Geometry: final body of the model. Coordinates: model frame, mm. A direction names the side the tool comes from. Round coordinates to 2 decimals unless told otherwise and drop trailing zeros. Order: outer loops, then holes, each group sorted by start corner. A loop starts at its lowest first (then second) coordinate and runs counter-clockwise, first axis right, second up. Notation, with made-up numbers: (77, 79.5) -> (132, 79.5) arc R23 cw to (132, 110.5) -> close; hole circle Ø3 at (62.5, 38.5). An arc over 180 degrees is marked (long way). Put each result on its own line as item: value.
```python
from build123d import *

# Parameters (mm, degrees)
SKETCH_W             = 14
SKETCH_H             = 6
PAD_DEPTH            = 4.8
THICKNESS_T          = -0.5
SKETCH001_W          = 8
SKETCH001_H          = 4.4
SKETCH001_W_2        = 1
SKETCH001_H_2        = 2
POCKET_DEPTH         = 0.5
SKETCH002_W          = 2.5
SKETCH002_H          = 1
SKETCH002_W_2        = 0.3
SKETCH002_H_2        = 0.3
POCKET001_DEPTH      = 7.001
POCKET001_DEPTH_BACK = 7.001
SKETCH004_W          = 1.5
SKETCH004_H          = 0.2
POCKET002_DEPTH      = 0.001
POCKET002_DEPTH_BACK = 4.801
LINEARPATTERN_COUNT  = 6
LINEARPATTERN_PITCH  = 2


with BuildPart() as part:
    # Sketch → Pad (new body)
    with BuildSketch(Plane.XY):
        with Locations((0, 3.4)):
            Rectangle(SKETCH_W, SKETCH_H)
    extrude(amount=PAD_DEPTH)

    # Thickness
    thickness_openings = [part.faces().sort_by_distance(p)[0] for p in [
        (0, 6.4, 2.4),
    ]]
    offset(amount=THICKNESS_T, openings=thickness_openings)

    # Sketch001 → Pocket (cut)
    with BuildSketch(Plane.XY.offset(4.8)):
        with Locations((0, 4.2)):
            Rectangle(SKETCH001_W, SKETCH001_H)
        with Locations((5.9, 3.8)):
            Rectangle(SKETCH001_W_2, SKETCH001_H_2)
        with Locations((-5.9, 3.8)):
            Rectangle(SKETCH001_W_2, SKETCH001_H_2)
    extrude(amount=-POCKET_DEPTH, mode=Mode.SUBTRACT)

    # Sketch002 → Pocket001 (cut, two sides)
    with BuildSketch(Plane.YZ) as pocket001_sk:
        with Locations((5.15, 3)):
            Rectangle(SKETCH002_W, SKETCH002_H)
        with Locations((0.95, 4.65)):
            Rectangle(SKETCH002_W_2, SKETCH002_H_2)
    extrude(amount=-POCKET001_DEPTH, mode=Mode.SUBTRACT)
    extrude(pocket001_sk.sketch, amount=POCKET001_DEPTH_BACK, mode=Mode.SUBTRACT)

    # Sketch004 → Pocket002 (cut, two sides)
    with BuildSketch(Plane.XY) as pocket002_sk:
        with Locations((-5, 0.5)):
            Rectangle(SKETCH004_W, SKETCH004_H)
    pocket002 = extrude(amount=-POCKET002_DEPTH, mode=Mode.SUBTRACT) + extrude(pocket002_sk.sketch, amount=POCKET002_DEPTH_BACK, mode=Mode.SUBTRACT)

    # LinearPattern: Pocket002 ×6
    with Locations(*[(i * LINEARPATTERN_PITCH, 0, 0) for i in range(1, LINEARPATTERN_COUNT)]):
        add(pocket002, mode=Mode.SUBTRACT)


solid = part.part
```
1. Cut plane C-C on y = 4.65. Return loops of the section in (x, z), and give its area (3 significant figures).
Ans:
outline: (-7, 0) -> (7, 0) -> (7, 2.5) -> (6.5, 2.5) -> (6.5, 0.5) -> (-6.5, 0.5) -> (-6.5, 2.5) -> (-7, 2.5) -> close; (-7, 3.5) -> (-6.5, 3.5) -> (-6.5, 4.3) -> (-6.4, 4.3) -> (-6.4, 4.8) -> (-7, 4.8) -> close; (-5.4, 4.3) -> (-4, 4.3) -> (-4, 4.8) -> (-5.4, 4.8) -> close; (4, 4.3) -> (5.4, 4.3) -> (5.4, 4.8) -> (4, 4.8) -> close; (6.4, 4.3) -> (6.5, 4.3) -> (6.5, 3.5) -> (7, 3.5) -> (7, 4.8) -> (6.4, 4.8) -> close
area: 11.8 mm²
2. Cut plane B-B on y = 3.75. Return loops of the section in (x, z).
Ans:
outline: (-7, 0) -> (7, 0) -> (7, 4.8) -> (6.4, 4.8) -> (6.4, 4.3) -> (6.5, 4.3) -> (6.5, 0.5) -> (-6.5, 0.5) -> (-6.5, 4.3) -> (-6.4, 4.3) -> (-6.4, 4.8) -> (-7, 4.8) -> close; (-5.4, 4.3) -> (-4, 4.3) -> (-4, 4.8) -> (-5.4, 4.8) -> close; (4, 4.3) -> (5.4, 4.3) -> (5.4, 4.8) -> (4, 4.8) -> close
3. Set-up query: faces 3 (the face through (6.5, 4, 2)), 4 (the face through (1, 0.6, 2)), 5 (the face through (0, 3, 0)). Return all of +Z, -Z, +X, -X, +Y, -Y with unobstructed straight access to the full face (end or side cutting, diameter ignored); none if empty.
Ans:
face 3: +Y
face 4: +Z, -Z, -Y
face 5: -Z, +X, -X, +Y, -Y
4. Draft query along X for faces 1 (the face through (6, 0.4, 2)), 2 (the face through (0, 4, 0.5)). Return one class per face: +X half, -X half, draft (parallel to the pull), parting line (faces both ways), or undercut.
Ans:
face 1: draft
face 2: undercut
5. Cut plane A-A on x = 6. Return loops of the section in (y, z).
Ans:
outline: (0.4, 0) -> (6.4, 0) -> (6.4, 0.5) -> (0.9, 0.5) -> (0.9, 4.3) -> (2.8, 4.3) -> (2.8, 4.8) -> (1.1, 4.8) -> (1.1, 4.5) -> (0.8, 4.5) -> (0.8, 4.8) -> (0.4, 4.8) -> close; (4.8, 4.3) -> (6.4, 4.3) -> (6.4, 4.8) -> (4.8, 4.8) -> close
6. Material intervals for probe 1 along X at (y, z) = (3, 4.35); probe 2 along X at (y, z) = (5.1, 0.8); probe 3 along Z at (x, y) = (-1.5, 0.95), sorted ascending.
Ans:
probe 1: -7 to -6.4, -5.4 to -4, 4 to 5.4, 6.4 to 7
probe 2: -7 to -6.5, 6.5 to 7
probe 3: 0 to 0.5, 4.3 to 4.5
7. Contact query for a flat-ended pin moving along its axis: P1, Ø1.5, axis at x = 4.5, z = 3, coming from the +Y side. Output: stop coordinate, or through.
Ans:
P1: y = 0.9
